Verification items for the finished model (mm, model axes). A direction names the side the tool comes from. Round coordinates to 2 decimals unless told otherwise and drop trailing zeros. Loops run counter-clockwise (first coordinate to the right, second up) from the corner with the lowest first, then second, coordinate; pieces in that order, holes last. Notation, with made-up numbers: M 84.25,-33 L 138.25,-33 A34 cw 138.25,-2 Z; hole C -20,-16.5 d8. An arc over 180 degrees is marked long. Answer as CSV lines item,"result".
```python
from build123d import *

# Parameters (mm, degrees)
SKETCH1_R           = 1.651
BOSS_EXTRUDE1_DEPTH = 9.525
CUT_EXTRUDE1_DEPTH  = 2.54


with BuildPart() as part:
    # Sketch1 → Boss-Extrude1 (new body)
    with BuildSketch(Plane.XY):
        Circle(SKETCH1_R)
    extrude(amount=BOSS_EXTRUDE1_DEPTH)

    # Sketch2 → Cut-Extrude1 (cut)
    with BuildSketch(Plane.XY.offset(9.525)):
        with BuildLine():
            Line((-0.889, 0), (-0.889, -0.381))
            Line((-0.889, -0.381), (0.7112, -0.381))
            Line((0.7112, -0.381), (0.889, -0.381))
            Line((0.889, -0.381), (0.889, 0))
            ThreePointArc((0.889, 0), (0, 0.889), (-0.889, 0))
        make_face()
    extrude(amount=-CUT_EXTRUDE1_DEPTH, mode=Mode.SUBTRACT)


solid = part.part
```
1) Set-up check for faces 1 (the flat face through (0, 0, 0)), 2 (the cylindrical face through (0.02, 0.89, 8.27)): record each of +Z, -Z, +X, -X, +Y, -Y from which the full face is reachable in a straight line by a thin tool's end or side.
Here are the results:
face 1,"-Z, +X, -X, +Y, -Y"
face 2,"+Z"
2) Section check C-C (z = 6). Record the cut outline in (x, y), plus the area to 3 significant figures.
Here are the results:
outline,"C 0,0 d3.3"
area,"8.56 mm^2"
3) Go/stop test with flat-tipped pins: pin 1 (0.6 mm diameter, centred on x = -0.5, y = 0, fed in from +Z) (3 decimals); pin 2 (1 mm diameter, centred on x = -0.5, y = -0.5, fed in from -Z). Record where each tip stops, or that it passes through.
Here are the results:
pin 1,"stops at z = 6.985"
pin 2,"stops at z = 0"
4) Section check D-D (y = -0.65). Record the cut outline in (x, z) (3 decimals).
Here are the results:
outline,"M -1.518,0 L 1.518,0 L 1.518,9.525 L -1.518,9.525 Z"
5) Section check B-B (x = 0). Record the cut outline in (y, z) (3 decimals).
Here are the results:
outline,"M -1.651,0 L 1.651,0 L 1.651,9.525 L 0.889,9.525 L 0.889,6.985 L -0.381,6.985 L -0.381,9.525 L -1.651,9.525 Z"
6) Draft check along Y on faces 3 (the flat face through (0, -1, 9.525)), 4 (the cylindrical face through (1.525, -0.632, 4.696)), 5 (the flat face through (0, -0.381, 8)). Enter one of: +Y half, -Y half, draft (parallel to the pull), parting line (faces both ways), or undercut.
Here are the results:
face 3,"draft"
face 4,"parting line"
face 5,"undercut"
7) Material ranges on probe 1 along Z at (x, y) = (-0.1, 0.4) (3 decimals); probe 2 along Y at (x, z) = (-0.75, 7.25); probe 3 along Y at (x, z) = (0.6, 8.75), recorded low to high.
Here are the results:
probe 1,"z = 0 to 6.985"
probe 2,"y = -1.47 to -0.38, 0.48 to 1.47"
probe 3,"y = -1.54 to -0.38, 0.66 to 1.54"
8) Section check A-A (z = 9.25). Record the cut outline in (x, y).
Here are the results:
outline,"C 0,0 d3.3; hole M -0.89,-0.38 L 0.89,-0.38 L 0.89,0 A0.89 ccw -0.89,0 Z"
